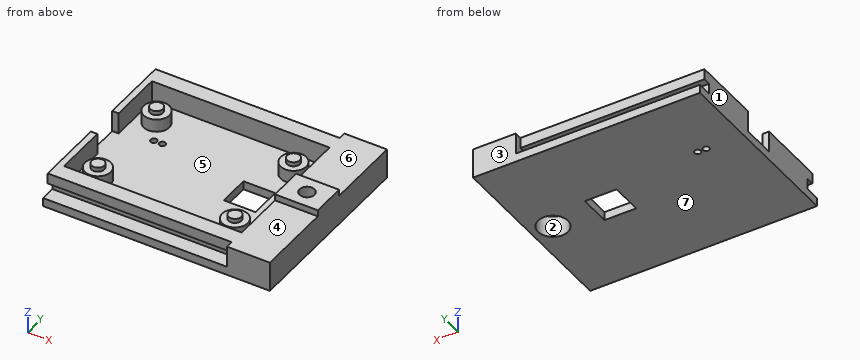
```python
from build123d import *

# Parameters (mm, degrees)
CROQUIS1_W              = 53
CROQUIS1_H              = 44
CROQUIS1_R              = 0.75
CROQUIS1_W_2            = 7.4
CROQUIS1_H_2            = 7.4
SALIENTE_EXTRUIR1_DEPTH = 2
CROQUIS4_R              = 1.5
SALIENTE_EXTRUIR3_DEPTH = 4
CORTAR_EXTRUIR1_REACH   = 40.484
CROQUIS5_R              = 1.75
CROQUIS6_R              = 1.75
CROQUIS6_W              = 41.5
CROQUIS6_H              = 33
SALIENTE_EXTRUIR4_DEPTH = 5
CROQUIS7_W              = 43
CROQUIS7_H              = 1.75
SALIENTE_EXTRUIR5_DEPTH = 2.5
CROQUIS8_W              = 1.5
CROQUIS8_H              = 8
CORTAR_EXTRUIR3_DEPTH   = 5
CROQUIS9_R              = 3.5
CORTAR_EXTRUIR4_DEPTH   = 5
CROQUIS10_R             = 3
SALIENTE_EXTRUIR6_DEPTH = 3
CROQUIS12_W             = 10
CROQUIS12_H             = 8
CROQUIS12_R             = 1.75
SALIENTE_EXTRUIR7_DEPTH = 1.5


with BuildPart() as part:
    # Croquis1 → Saliente-Extruir1 (new body)
    with BuildSketch(Plane.XY):
        with Locations((4.5, 0)):
            Rectangle(CROQUIS1_W, CROQUIS1_H)
        with Locations((-13.3084, 5.6686)):
            Circle(CROQUIS1_R, mode=Mode.SUBTRACT)
        with Locations((-11.3084, 5.6686)):
            Circle(CROQUIS1_R, mode=Mode.SUBTRACT)
        with Locations((12.55, 0)):
            Rectangle(CROQUIS1_W_2, CROQUIS1_H_2, mode=Mode.SUBTRACT)
    extrude(amount=SALIENTE_EXTRUIR1_DEPTH)

    # Croquis4 → Saliente-Extruir3 (add)
    with BuildSketch(Plane.XY.offset(2)):
        with Locations((-16, -11)):
            Circle(CROQUIS4_R)
        with Locations((16, -11)):
            Circle(CROQUIS4_R)
        with Locations((16, 11)):
            Circle(CROQUIS4_R)
        with Locations((-16, 11)):
            Circle(CROQUIS4_R)
    extrude(amount=SALIENTE_EXTRUIR3_DEPTH)

    # Croquis5 → Cortar-Extruir1 (cut, up to next)
    with BuildSketch(Plane(origin=(0, 0, 0), x_dir=(-1, 0, 0), z_dir=(0, 0, -1)), mode=Mode.PRIVATE) as cortar_extruir1_sk1:
        with Locations((-26, 0)):
            Circle(CROQUIS5_R)
    cortar_extruir1_tool1 = extrude(cortar_extruir1_sk1.sketch, amount=-CORTAR_EXTRUIR1_REACH, mode=Mode.PRIVATE) & part.part
    add(cortar_extruir1_tool1.solids().sort_by_distance((26, 0, 0))[0], mode=Mode.SUBTRACT)

    # Croquis6 → Saliente-Extruir4 (add)
    with BuildSketch(Plane.XY.offset(2)):
        Polygon((-22, -18.5), (21, -18.5), (21, -22), (31, -22), (31, 22), (21, 22), (21, 18.5), (-22, 18.5), align=None)
        with Locations(Location((26, 0, 0), (0, 0, 180))):
            Circle(CROQUIS6_R, mode=Mode.SUBTRACT)
        with Locations((0.25, 0)):
            Rectangle(CROQUIS6_W, CROQUIS6_H, mode=Mode.SUBTRACT)
    extrude(amount=SALIENTE_EXTRUIR4_DEPTH)

    # Croquis7 → Saliente-Extruir5 (add)
    with BuildSketch(Plane.XY.offset(7)):
        with Locations((-0.5, 19.375)):
            Rectangle(CROQUIS7_W, CROQUIS7_H)
        with Locations((-0.5, -19.375)):
            Rectangle(CROQUIS7_W, CROQUIS7_H)
    extrude(amount=-SALIENTE_EXTRUIR5_DEPTH)

    # Croquis8 → Cortar-Extruir3 (cut)
    with BuildSketch(Plane.XY.offset(7)):
        with Locations((-21.25, 0)):
            Rectangle(CROQUIS8_W, CROQUIS8_H)
    extrude(amount=-CORTAR_EXTRUIR3_DEPTH, mode=Mode.SUBTRACT)

    # Croquis9 → Cortar-Extruir4 (cut)
    with BuildSketch(Plane(origin=(0, 0, 0), x_dir=(-1, 0, 0), z_dir=(0, 0, -1))):
        with Locations((-26, 0)):
            Circle(CROQUIS9_R)
    extrude(amount=-CORTAR_EXTRUIR4_DEPTH, mode=Mode.SUBTRACT)

    # Croquis10 → Saliente-Extruir6 (add)
    with BuildSketch(Plane.XY.offset(2)):
        with Locations((-16, 11)):
            Circle(CROQUIS10_R)
        with Locations((16, 11)):
            Circle(CROQUIS10_R)
        with Locations((16, -11)):
            Circle(CROQUIS10_R)
        with Locations((-16, -11)):
            Circle(CROQUIS10_R)
    extrude(amount=SALIENTE_EXTRUIR6_DEPTH)

    # Croquis12 → Saliente-Extruir7 (add)
    with BuildSketch(Plane.XY.offset(7)):
        with Locations((26, 0)):
            Rectangle(CROQUIS12_W, CROQUIS12_H)
        with Locations(Location((26, 0, 0), (0, 0, 180))):
            Circle(CROQUIS12_R, mode=Mode.SUBTRACT)
    extrude(amount=SALIENTE_EXTRUIR7_DEPTH)


solid = part.part
```
Here's how the part is built. I have some questions about the finished solid (model axes, mm). Face numbers are marked on the shaded views. A direction names the side the tool comes from. Give positions to 0.01 mm unless a question says otherwise; leave off trailing zeros. Order: outer loops, then holes, each group sorted by start corner. A loop starts at its lowest first (then second) coordinate and runs counter-clockwise, first axis right, second up. Notation, with made-up numbers: (32.5, 71.5) - (60.5, 71.5) arc R30 cw to (60.5, 102.5) - close; hole circle Ø10 at (77, 4). An arc over 180 degrees is marked (long way). Answer as a JSON object with one key per item and string values. Group by question number.
Item 1: If we mould it in two halves opening along X, with no side actions, what happens to the marked faces 1, 2 and 3? For each: pulls with the +X half, pulls with the -X half, needs draft (parallel to the pull), parting line crosses it, or undercut.
Item 2: If we section it at A-A on x = 26: Please give me the cut outline in (y, z).
Item 3: If we section it at C-C on y = 0: Please give me the cut outline in (x, z), and give its area (3 significant figures).
Item 4: Which directions (+Z, -Z, +X, -X, +Y, -Y) give clear straight access to the entire face, cutting with the end or side of a thin tool? Please do the marked faces 4, 5, 6 and 7.
Item 5: For P1, Ø5.5, axis at x = 26.5, y = -0.5, coming from the -Z side; P2, Ø2, axis at x = 11.5, z = 5.5, coming from the -Y side; P3, Ø2, axis at x = -10.5, z = 7.5, coming from the +Y side; P4, Ø1.4, axis at x = -13.31, y = 5.67, coming from the -Z side, each with a flat end and sliding along its axis, tell me the tip position at first contact or that it passes through.
Item 6: If we section it at B-B on z = 3.5: Please give me the cut outline in (x, y).
Item 7: Please list where these lines run through material, in increasing order: probe 1 along Y at (x, z) = (14, 1); probe 2 along Y at (x, z) = (-4, 5.75); probe 3 along X at (y, z) = (10.5, 5.25).
Item 8: If we section it at D-D on y = 11: Please give me the cut outline in (x, z), and give its area (4 significant figures).
Result set:
{
 "1": {"face 1": "pulls with the -X half", "face 2": "undercut", "face 3": "needs draft"},
 "2": {"outline": "(-22, 0) - (-3.5, 0) - (-3.5, 5) - (-1.75, 5) - (-1.75, 8.5) - (-4, 8.5) - (-4, 7) - (-22, 7) - close; (1.75, 5) - (3.5, 5) - (3.5, 0) - (22, 0) - (22, 7) - (4, 7) - (4, 8.5) - (1.75, 8.5) - close"},
 "3": {"outline": "(-22, 0) - (8.85, 0) - (8.85, 2) - (-22, 2) - close; (16.25, 0) - (22.5, 0) - (22.5, 5) - (24.25, 5) - (24.25, 8.5) - (21, 8.5) - (21, 2) - (16.25, 2) - close; (27.75, 5) - (29.5, 5) - (29.5, 0) - (31, 0) - (31, 8.5) - (27.75, 8.5) - close", "area": "109 mm²"},
 "4": {"face 4": "+Z, +X, -X, -Y", "face 5": "+Z", "face 6": "+Z, +X, -X, +Y", "face 7": "-Z, +X, -X, +Y, -Y"},
 "5": {"P1": "z = 5", "P2": "y = -20.25", "P3": "y = 20.25", "P4": "through"},
 "6": {"outline": "(-22, -18.5) - (21, -18.5) - (21, -22) - (31, -22) - (31, 22) - (21, 22) - (21, 18.5) - (-22, 18.5) - (-22, 4) - (-20.5, 4) - (-20.5, 16.5) - (21, 16.5) - (21, -16.5) - (-20.5, -16.5) - (-20.5, -4) - (-22, -4) - close; circle Ø6 at (-16, -11); circle Ø6 at (-16, 11); circle Ø6 at (16, -11); circle Ø6 at (16, 11); hole circle Ø7 at (26, 0)"},
 "7": {"probe 1": "-22 to -3.7, 3.7 to 22", "probe 2": "-20.25 to -16.5, 16.5 to 20.25", "probe 3": "-22 to -20.5, -17.41 to -14.59, 14.59 to 17.41, 21 to 31"},
 "8": {"outline": "(-22, 0) - (31, 0) - (31, 7) - (21, 7) - (21, 2) - (19, 2) - (19, 5) - (17.5, 5) - (17.5, 6) - (14.5, 6) - (14.5, 5) - (13, 5) - (13, 2) - (-13, 2) - (-13, 5) - (-14.5, 5) - (-14.5, 6) - (-17.5, 6) - (-17.5, 5) - (-19, 5) - (-19, 2) - (-20.5, 2) - (-20.5, 7) - (-22, 7) - close", "area": "205.5 mm²"}
}
